Check sheet for the modelled part. Datum: model origin and axes. Units: mm. Face numbers are marked on the shaded views. A direction names the side the tool comes from. Give positions to 0.01 mm unless a question says otherwise; leave off trailing zeros. Order: outer loops, then holes, each group sorted by start corner. A loop starts at its lowest first (then second) coordinate and runs counter-clockwise, first axis right, second up. Notation, with made-up numbers: M 26,82.5 L 73,82.5 A27 cw 73,104.5 Z; hole C -20.75,82 d7. An arc over 180 degrees is marked long. Answer in a Markdown table with one row per item. Add a question column.
from build123d import *

# Parameters (mm, degrees)
F0_W      = 145
F0_H      = 72
F1_DEPTH  = 90
F2_W      = 109
F2_H      = 65
F3_DEPTH  = 90
F5_DEPTH  = 25.4
F6_W      = 50
F6_H      = 6
F7_DEPTH  = 72
F9_DEPTH  = 12
F10_R     = 18
F11_DEPTH = 24


with BuildPart() as f1:
    # F0 (on Top) → F1 (new body)
    with BuildSketch(Plane.XY):
        with Locations((-72.5, 36)):
            Rectangle(F0_W, F0_H)
    extrude(amount=F1_DEPTH)

    # F2 (on face) → F3 (cut)
    with BuildSketch(Plane.XZ):
        with Locations((-54.5, 57.5)):
            Rectangle(F2_W, F2_H)
    extrude(amount=-F3_DEPTH, mode=Mode.SUBTRACT)

    # F4 (on face) → F5 (cut)
    with BuildSketch(Plane.XY.offset(25)):
        with BuildLine():
            Line((-50, 19.744541496), (0, 19.744541496))
            Line((0, 19.744541496), (0, 43.744541496))
            Line((0, 43.744541496), (-50, 43.744541496))
            ThreePointArc((-50, 43.744541496), (-62, 31.744541496), (-50, 19.744541496))
        make_face()
    extrude(amount=-F5_DEPTH, mode=Mode.SUBTRACT)

    # F6 (on face) → F7 (cut)
    with BuildSketch(Plane(origin=(-145, 0, 0), x_dir=(0, -1, 0), z_dir=(-1, 0, 0))):
        with Locations((-25, 3)):
            Rectangle(F6_W, F6_H)
    extrude(amount=-F7_DEPTH, mode=Mode.SUBTRACT)

    # F8 (on face) → F9 (cut)
    with BuildSketch(Plane(origin=(-145, 0, 0), x_dir=(0, -1, 0), z_dir=(-1, 0, 0))):
        with BuildLine():
            ThreePointArc((-62.9122615735, 30), (-68.3769952744, 48), (-62.9122615735, 66))
            Line((-62.9122615735, 66), (-72, 66))
            Line((-72, 66), (-72, 30))
            Line((-72, 30), (-62.9122615735, 30))
        make_face()
        with BuildLine():
            Line((-62.9122615735, 66), (-9.0877384265, 66))
            ThreePointArc((-9.0877384265, 66), (-36, 80.3769952744), (-62.9122615735, 66))
        make_face()
        with BuildLine():
            ThreePointArc((-9.0877384265, 66), (-5.0192964187, 57.4056274966), (-3.6230047256, 48))
            ThreePointArc((-3.6230047256, 48), (-5.0192964187, 38.5943725034), (-9.0877384265, 30))
            Line((-9.0877384265, 30), (0, 30))
            Line((0, 30), (0, 66))
            Line((0, 66), (-9.0877384265, 66))
        make_face()
        with BuildLine():
            ThreePointArc((-62.9122615735, 30), (-36, 15.6230047256), (-9.0877384265, 30))
            Line((-9.0877384265, 30), (-62.9122615735, 30))
        make_face()
        with BuildLine():
            ThreePointArc((-9.0877384265, 30), (-5.0192964187, 38.5943725034), (-3.6230047256, 48))
            ThreePointArc((-3.6230047256, 48), (-5.0192964187, 57.4056274966), (-9.0877384265, 66))
            Line((-9.0877384265, 66), (-62.9122615735, 66))
            ThreePointArc((-62.9122615735, 66), (-68.3769952744, 48), (-62.9122615735, 30))
            Line((-62.9122615735, 30), (-9.0877384265, 30))
        make_face()
    extrude(amount=-F9_DEPTH, mode=Mode.SUBTRACT)

    # F10 (on face) → F11 (cut, through all)
    with BuildSketch(Plane(origin=(-133, 0, 0), x_dir=(0, -1, 0), z_dir=(-1, 0, 0))):
        with Locations((-36, 48)):
            Circle(F10_R)
    extrude(amount=-F11_DEPTH, mode=Mode.SUBTRACT)


solid = f1.part
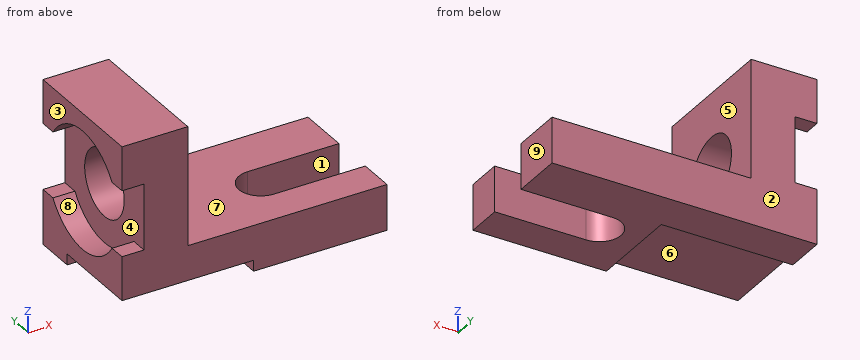
Q1. Cross-section at C-C (y = 36). Record the boundary of the cut face in (x, z).
Q2. Cross-section at A-A (x = -116.5). Record the boundary of the cut face in (y, z), and give its area (3 significant figures).
Q3. Cross-section at B-B (z = 48). Record the boundary of the cut face in (x, y).
Q4. Tool access check on the marked faces 1, 2, 3, 4 and 5. Record the directions out of +Z, -Z, +X, -X, +Y, -Y that give a thin tool (end or side, any length) a straight path to the whole face; none if there is none.
Q5. Draft check along Z on the marked faces 6, 7, 8 and 9. Enter one of: pulls with the +Z half, pulls with the -Z half, needs draft (parallel to the pull), parting line crosses it, or undercut.
Q6. Go/stop test with flat-tipped pins: pin 1 (2.5 mm diameter, centred on x = -137.5, y = 6, fed in from -Z); pin 2 (1.8 mm diameter, centred on y = 23.5, z = 2, fed in from -X); pin 3 (6 mm diameter, centred on x = -38, y = 42, fed in from +Z). Record where each tip stops, or that it passes through.
Q7. Thickness scan on probe 1 along Y at (x, z) = (-7, 15); probe 2 along Z at (x, y) = (-121.75, 36); probe 3 along X at (y, z) = (7, 65). Record the ranges inside material, lowest first.
Q8. Cross-section at D-D (x = -76). Record the boundary of the cut face in (y, z).
Values follow:
| question | item | result |
|---|---|---|
| 1 | outline | M -145,6 L -73,6 L -73,0 L -61.22,0 L -61.22,25 L -109,25 L -109,30 L -133,30 L -133,15.62 L -145,15.62 Z; M -145,80.38 L -133,80.38 L -133,66 L -109,66 L -109,90 L -145,90 Z |
| 2 | outline | M 0,6 L 50,6 L 50,0 L 72,0 L 72,90 L 0,90 Z; hole C 36,48 d36 |
| 2 | area | 5,160 mm² |
| 3 | outline | M -133,0 L -109,0 L -109,18 L -133,18 Z; M -133,54 L -109,54 L -109,72 L -133,72 Z |
| 4 | face 1 | +Z, -Z, +X |
| 4 | face 2 | +Z, -Z, +X, -X, +Y |
| 4 | face 3 | +Z, -Z, -X, +Y, -Y |
| 4 | face 4 | -X |
| 4 | face 5 | +Z, +X, +Y, -Y |
| 5 | face 6 | pulls with the -Z half |
| 5 | face 7 | pulls with the +Z half |
| 5 | face 8 | undercut |
| 5 | face 9 | needs draft |
| 6 | pin 1 | z = 6 |
| 6 | pin 2 | x = -73 |
| 6 | pin 3 | z = 25 |
| 7 | probe 1 | 0 to 19.74, 43.74 to 72 |
| 7 | probe 2 | 6 to 30, 66 to 90 |
| 7 | probe 3 | -133 to -109 |
| 8 | outline | M 0,6 L 50,6 L 50,0 L 72,0 L 72,25 L 0,25 Z |
